```python
from build123d import *

# Parameters (mm, degrees)
SKETCH1_R               = 22
BOSS_EXTRUDE1_DEPTH     = 4.5
SKETCH2_R               = 20.8
SKETCH2_R_2             = 19.84
BOSS_EXTRUDE2_DEPTH     = 1.2
SKETCH3_R               = 18
CUT_EXTRUDE1_DEPTH      = 32.630523233
CUT_EXTRUDE2_DEPTH      = 32.436443819
CUT_EXTRUDE2_DEPTH_BACK = 3.9
CUT_EXTRUDE3_DEPTH      = 32.436443819
CUT_EXTRUDE3_DEPTH_BACK = 3.1
FILLET1_R               = 2
FILLET2_R               = 1
CUT_EXTRUDE4_DEPTH      = 32.436443819


with BuildPart() as part:
    # Sketch1 → Boss-Extrude1 (new body)
    with BuildSketch(Plane(origin=(0, 0, 0), x_dir=(1, 0, 0), z_dir=(0, 1, 0))):
        with Locations(Location((0, 0, 0), (0, 0, 270))):
            Circle(SKETCH1_R)
    extrude(amount=BOSS_EXTRUDE1_DEPTH)

    # Sketch2 → Boss-Extrude2 (add)
    with BuildSketch(Plane.XZ):
        with Locations(Location((0, 0, 0), (0, 0, 90))):
            Circle(SKETCH2_R)
        with Locations(Location((0, 0, 0), (0, 0, 270))):
            Circle(SKETCH2_R_2, mode=Mode.SUBTRACT)
    extrude(amount=BOSS_EXTRUDE2_DEPTH)

    # Sketch3 → Cut-Extrude1 (cut, through all)
    with BuildSketch(Plane(origin=(0, 4.5, 0), x_dir=(1, 0, 0), z_dir=(0, 1, 0))):
        with Locations(Location((0, 0, 0), (0, 0, 270))):
            Circle(SKETCH3_R)
    extrude(amount=-CUT_EXTRUDE1_DEPTH, mode=Mode.SUBTRACT)

    # Sketch4 → Cut-Extrude2 (cut, two sides: drawn at the far end of the back side and taken through both)
    with BuildSketch(Plane.XZ.offset(-CUT_EXTRUDE2_DEPTH_BACK)):
        with BuildLine():
            Line((-13.481253655, -13.88086092), (-7.85, -19.35))
            Line((-7.85, -19.35), (7.85, -19.35))
            Line((7.85, -19.35), (13.481253655, -13.88086092))
            ThreePointArc((13.481253655, -13.88086092), (0, 19.35), (-13.481253655, -13.88086092))
        make_face()
    extrude(amount=CUT_EXTRUDE2_DEPTH + CUT_EXTRUDE2_DEPTH_BACK, mode=Mode.SUBTRACT)

    # Sketch5 → Cut-Extrude3 (cut, two sides: drawn at the far end of the back side and taken through both)
    with BuildSketch(Plane.XZ.offset(-CUT_EXTRUDE3_DEPTH_BACK)):
        Polygon((-6.6, -20.85), (6.6, -20.85), (7.25, -19.35), (-7.25, -19.35), align=None)
    extrude(amount=CUT_EXTRUDE3_DEPTH + CUT_EXTRUDE3_DEPTH_BACK, mode=Mode.SUBTRACT)

    # Fillet1
    fillet1_edges = [part.edges().sort_by_distance(p)[0] for p in [
        (0, 4.5, -22),
    ]]
    fillet(fillet1_edges, radius=FILLET1_R)

    # Fillet2
    fillet2_edges = [part.edges().sort_by_distance(p)[0] for p in [
        (0, 3.1, -20.85),
    ]]
    fillet(fillet2_edges, radius=FILLET2_R)

    # Sketch6 → Cut-Extrude4 (cut, through all)
    with BuildSketch(Plane.XZ):
        with BuildLine():
            Line((7.25, -19.35), (7.174883279, -19.523346279))
            ThreePointArc((7.174883279, -19.523346279), (7.402968696, -19.438005414), (7.630039318, -19.35))
            Line((7.630039318, -19.35), (7.25, -19.35))
        make_face()
        with BuildLine():
            Line((-7.174883279, -19.523346279), (-7.25, -19.35))
            Line((-7.25, -19.35), (-7.630039318, -19.35))
            ThreePointArc((-7.630039318, -19.35), (-7.402968696, -19.438005414), (-7.174883279, -19.523346279))
        make_face()
    extrude(amount=CUT_EXTRUDE4_DEPTH, mode=Mode.SUBTRACT)


solid = part.part
```
Model file for the job. Use its own axes, mm. A direction names the side the tool comes from. Give positions to 0.01 mm unless a question says otherwise; leave off trailing zeros. Order: outer loops, then holes, each group sorted by start corner. A loop starts at its lowest first (then second) coordinate and runs counter-clockwise, first axis right, second up.
1) Saw through at B-B, the plane x = 0. Write the cut outline in (y, z), then the cut area to 3 significant figures.
2) Wall check: probe 1 along X at (y, z) = (2.2, 0); probe 2 along X at (y, z) = (0.75, -19); probe 3 along Z at (x, y) = (-9, 3.45). Give the ranges that are in metal, low to high.
3) Pin check, flat tips, straight feed: pin 1 (22 mm diameter, centred on x = 3, z = 7, fed in from -Y); pin 2 (0.6 mm diameter, centred on x = 3, y = 1.5, fed in from +Z); pin 3 (1 mm diameter, centred on y = 0, z = 9.5, fed in from -X). Stop position of each tip, or through.
4) Saw through at C-C, the plane y = 1.45. Write the cut outline in (x, z), then the cut area to 3 significant figures.
5) 3-axis set-ups, long thin cutter, end or side, ignore diameter. For faces 4 (the flat face through (3, 4.5, -18)), 5 (the cylindrical face through (0.64, 1.98, 19.34)): which of +Z, -Z, +X, -X, +Y, -Y reach the whole face in a straight line?
6) Mould opens along X. For faces 1 (the flat face through (11.4, 3.9, -14.2)), 2 (the cylindrical face through (-21.477, 1.232, -4.769)), 3 (the flat face through (0, -1.2, 20)) say: +X half, -X half, draft (parallel to the pull), parting line (faces both ways), or undercut.
7) Saw through at A-A, the plane z = 0. Write the cut outline in (x, y), then the cut area to 3 significant figures.
Computed:
1. outline: (-1.2, 19.84) - (0, 19.84) - (0, 19.35) - (3.9, 19.35) - (3.9, 18) - (4.5, 18) - (4.5, 20) arc R2 ccw to (2.5, 22) - (0, 22) - (0, 20.8) - (-1.2, 20.8) - close; (0, -22) - (2.5, -22) arc R2 ccw to (4.5, -20) - (4.5, -18) - (3.9, -18) - (3.9, -19.35) - (3.1, -19.35) - (3.1, -19.85) arc R1 cw to (2.1, -20.85) - (0, -20.85) - close
1. area: 20.5 mm2
2. probe 1: x = -22 to -19.35, 19.35 to 22
2. probe 2: x = -11.09 to -8.21, 8.21 to 11.09
2. probe 3: z = -19.81 to -18.23, 17.13 to 19.81
3. pin 1: stops at y = 3.9
3. pin 2: stops at z = 21.83
3. pin 3: stops at x = -20.07
4. outline: circle Ø44 at (0, 0); hole (-13.48, -13.88) - (-7.85, -19.35) - (-7.25, -19.35) - (-6.6, -20.85) - (6.6, -20.85) - (7.25, -19.35) - (7.85, -19.35) - (13.48, -13.88) arc R19.35 ccw (long way) to start
4. area: 308 mm2
5. face 4: +Z, -Z, +X, -X, +Y
5. face 5: -Y
6. face 1: undercut
6. face 2: parting line
6. face 3: draft
7. outline: (-22, 0) - (-20.8, 0) - (-20.8, -1.2) - (-19.84, -1.2) - (-19.84, 0) - (-19.35, 0) - (-19.35, 3.9) - (-18, 3.9) - (-18, 4.5) - (-20, 4.5) arc R2 ccw to (-22, 2.5) - close; (18, 3.9) - (19.35, 3.9) - (19.35, 0) - (19.84, 0) - (19.84, -1.2) - (20.8, -1.2) - (20.8, 0) - (22, 0) - (22, 2.5) arc R2 ccw to (20, 4.5) - (18, 4.5) - close
7. area: 26.1 mm2
